from build123d import *

# Parameters (mm, degrees)
SKETCH1_R               = 3.175
SKETCH1_R_2             = 11
BOSS_EXTRUDE1_DEPTH     = 6.35
CUT_EXTRUDE1_REACH      = 122.068
CUT_EXTRUDE1_END_RADIUS = 11
SKETCH2_R               = 1.1303
SKETCH3_W               = 25.4
SKETCH3_H               = 6.35
SKETCH3_W_2             = 6.35
BOSS_EXTRUDE2_DEPTH     = 4.7625
FILLET3_R               = 2


with BuildPart() as part:
    # Sketch1 → Boss-Extrude1 (new body)
    with BuildSketch(Plane.XY):
        with BuildLine():
            Line((-25.4, -12.7), (-25.4, 12.7))
            Line((-25.4, 12.7), (45.199208724, 12.7))
            Line((45.199208724, 12.7), (74.463216326, -5.044542368))
            ThreePointArc((74.463216326, -5.044542368), (88.585378941, -10.82071629), (91.444603929, -25.808194216))
            Line((91.444603929, -25.808194216), (87.555933896, -32.221324916))
            ThreePointArc((87.555933896, -32.221324916), (72.944550454, -36.615313538), (61.293587146, -26.763678338))
            Line((61.293587146, -26.763678338), (38.1, -12.7))
            Line((38.1, -12.7), (-25.4, -12.7))
        make_face()
        Circle(SKETCH1_R, mode=Mode.SUBTRACT)
        with Locations((76.2, -20.95)):
            Circle(SKETCH1_R_2, mode=Mode.SUBTRACT)
    extrude(amount=BOSS_EXTRUDE1_DEPTH)

    # Cut-Extrude1: up to this cylinder (the profile starts outside it)
    cut_extrude1_end = Plane(origin=(76.2, -20.95, 3.175), z_dir=(0, 0, -1)) * Cylinder(CUT_EXTRUDE1_END_RADIUS, 267.136, mode=Mode.PRIVATE)
    # Sketch2 → Cut-Extrude1 (cut, up to the surface)
    with BuildSketch(Plane(origin=(78.303556067, -47.480194346, 0), x_dir=(0, 0, -1), z_dir=(0.8550840932924629, -0.5184893377864258, 0)), mode=Mode.PRIVATE) as cut_extrude1_sk1:
        with Locations(Location((-3.175, 21.594875785, 0), (0, 0, 90))):
            Circle(SKETCH2_R)
    cut_extrude1_tool1 = extrude(cut_extrude1_sk1.sketch, amount=-CUT_EXTRUDE1_REACH, mode=Mode.PRIVATE) - cut_extrude1_end
    add(cut_extrude1_tool1.solids().sort_by_distance((89.500269, -29.01476, 3.175))[0], mode=Mode.SUBTRACT)

    # Sketch3 → Boss-Extrude2 (add)
    with BuildSketch(Plane.XY):
        with Locations((20.6375, 0)):
            Rectangle(SKETCH3_W, SKETCH3_H)
        with Locations((-15.875, 0)):
            Rectangle(SKETCH3_W_2, SKETCH3_H)
    extrude(amount=-BOSS_EXTRUDE2_DEPTH)

    # Fillet3
    fillet3_edges = [part.edges().sort_by_distance(p)[0] for p in [
        (-25.4, -12.7, 3.175),
        (-25.4, 12.7, 3.175),
        (45.199208724, 12.7, 3.175),
        (38.1, -12.7, 3.175),
        (33.3375, 3.175, -2.38125),
        (33.3375, -3.175, -2.38125),
        (7.9375, -3.175, -2.38125),
        (7.9375, 3.175, -2.38125),
        (-12.7, 3.175, -2.38125),
        (-12.7, -3.175, -2.38125),
        (-19.05, -3.175, -2.38125),
        (-19.05, 3.175, -2.38125),
    ]]
    fillet(fillet3_edges, radius=FILLET3_R)


solid = part.part
Check sheet for the modelled part. Datum: model origin and axes. Units: mm. A direction names the side the tool comes from. Round coordinates to 2 decimals unless told otherwise and drop trailing zeros. Order: outer loops, then holes, each group sorted by start corner. A loop starts at its lowest first (then second) coordinate and runs counter-clockwise, first axis right, second up. Notation, with made-up numbers: M 10,-5 L 25,-5 A29 cw 25,30 Z; hole C 45.5,-17.75 d4. An arc over 180 degrees is marked long. One line per item, written item: value. Start each with the question number.
1. Access from +Z, -Z, +X, -X, +Y, -Y to the whole of each face (thin tool, end or side, straight path). Record for faces 5 (the cylindrical face through (32.77, -2.57, -2.41)), 6 (the flat face through (7, -12.7, 3)), 7 (the cylindrical face through (8.508, 2.574, -2.415)).
2. Section check D-D on x = 0. Enter the section's corners in (y, z) (3 decimals).
3. Scan lines: line 1 along Y through (x, z) = (0, 5.25) (3 decimals); line 2 along Z through (x, y) = (56.5, -22); line 3 along Y through (x, z) = (76.2, 1.75). Record each from-to range of solid material in increasing order.
4. Release check for a two-part mould opening along X. For faces 1 (the cylindrical face through (-0.69, -3.1, 3.13)), 2 (the flat face through (-19.05, 0, -2)), 3 (the flat face through (89.527, -28.97, 1.719)), 4 (the cylindrical face through (87.123, -28.548, 3.939)) record: released by +X, released by -X, zero draft, split by the parting line, or undercut.
5. Gauge pin test, flat ends, axial feed: P1, Ø2.5, axis at y = 0, z = -1.5, coming from the +X side; P2, Ø4, axis at x = 0, y = 0, coming from the +Z side; P3, Ø1.9, axis at x = 4, z = 3, coming from the -Y side; P4, Ø1.2, axis at x = -16, z = -3, coming from the +Y side (3 decimals). Record the tip position at first contact, or that the pin passes through.
6. Section check A-A on x = 76.2. Enter the section's corners in (y, z).
Results found:
1. face 5: -Z, +X, -Y
1. face 6: +Z, -Z, -X, -Y
1. face 7: -Z, +Y
2. outline: M -12.7,0 L -3.175,0 L -3.175,6.35 L -12.7,6.35 Z; M 3.175,0 L 12.7,0 L 12.7,6.35 L 3.175,6.35 Z
3. line 1: -12.7 to -3.175, 3.175 to 12.7
3. line 2: 0 to 6.35
3. line 3: -36.95 to -31.95, -9.95 to -4.95
4. face 1: undercut
4. face 2: released by -X
4. face 3: released by +X
4. face 4: undercut
5. P1: x = 33.34
5. P2: through
5. P3: y = -12.7
5. P4: y = 3.175
6. outline: M -36.95,0 L -31.95,0 L -31.95,6.35 L -36.95,6.35 Z; M -9.95,0 L -4.95,0 L -4.95,6.35 L -9.95,6.35 Z
